For this review, take the finished solid that the model builds, in its own axes (mm). A direction names the side the tool comes from. Round coordinates to 2 decimals unless told otherwise and drop trailing zeros. Write each loop counter-clockwise with the first axis right and the second up, starting at its lowest first coordinate (ties: lowest second). Pieces come first, ordered by that corner, then holes. Notation, with made-up numbers: M -30,58 L 13,58 A20 cw 13,63 Z; hole C -40,56.5 d11. An arc over 180 degrees is marked long. Write each question's results on one line, items separated by ' | '. Start each with the question number.
```python
from build123d import *

# Parameters (mm, degrees)
SKETCH_1_W          = 250
SKETCH_1_H          = 156
SKETCH_1_W_2        = 226
SKETCH_1_H_2        = 128
EXTRUDE_1_DEPTH     = 8
SKETCH_2_W          = 235.5
SKETCH_2_H          = 139.5
CUT_EXTRUDE_3_DEPTH = 6
SKETCH_11_W         = 250
SKETCH_11_H         = 8
EXTRUDE_3_DEPTH     = 3.75
CUT_EXTRUDE_4_DEPTH = 10
SKETCH_13_R         = 1.5
CUT_EXTRUDE_5_DEPTH = 10
SKETCH_14_R         = 3
CUT_EXTRUDE_6_DEPTH = 2


with BuildPart() as part:
    # 草图1 → 凸台-拉伸1 (new body)
    with BuildSketch(Plane(origin=(0, 0, 0), x_dir=(1, 0, 0), z_dir=(0, 1, 0))):
        with Locations((25.659327926, -14.898030127)):
            Rectangle(SKETCH_1_W, SKETCH_1_H)
        with Locations((25.659327926, -14.898030127)):
            Rectangle(SKETCH_1_W_2, SKETCH_1_H_2, mode=Mode.SUBTRACT)
    extrude(amount=EXTRUDE_1_DEPTH)

    # 草图2 → 切除-拉伸3 (cut)
    with BuildSketch(Plane.XZ):
        with Locations((24.659327926, 12.898030127)):
            Rectangle(SKETCH_2_W, SKETCH_2_H)
    extrude(amount=-CUT_EXTRUDE_3_DEPTH, mode=Mode.SUBTRACT)

    # 草图11 → 凸台-拉伸3 (add)
    with BuildSketch(Plane(origin=(0, 0, -63.101969873), x_dir=(-1, 0, 0), z_dir=(0, 0, -1))):
        with Locations((-25.659327926, 4)):
            Rectangle(SKETCH_11_W, SKETCH_11_H)
    extrude(amount=EXTRUDE_3_DEPTH)

    # 草图12 → 切除-拉伸4 (cut)
    with BuildSketch(Plane.XZ):
        with BuildLine():
            Line((-89.340672074, 92.898030127), (-99.340672074, 92.898030127))
            Line((-99.340672074, 92.898030127), (-99.340672074, 82.898030127))
            ThreePointArc((-99.340672074, 82.898030127), (-96.411739886, 89.969097939), (-89.340672074, 92.898030127))
        make_face()
        with BuildLine():
            Line((-99.340672074, -56.851969873), (-99.340672074, -66.851969873))
            Line((-99.340672074, -66.851969873), (-89.340672074, -66.851969873))
            ThreePointArc((-89.340672074, -66.851969873), (-96.411739886, -63.923037684), (-99.340672074, -56.851969873))
        make_face()
        with BuildLine():
            Line((140.659327926, -66.851969873), (150.659327926, -66.851969873))
            Line((150.659327926, -66.851969873), (150.659327926, -56.851969873))
            ThreePointArc((150.659327926, -56.851969873), (147.730395738, -63.923037684), (140.659327926, -66.851969873))
        make_face()
        with BuildLine():
            Line((150.659327926, 82.898030127), (150.659327926, 92.898030127))
            Line((150.659327926, 92.898030127), (140.659327926, 92.898030127))
            ThreePointArc((140.659327926, 92.898030127), (147.730395738, 89.969097939), (150.659327926, 82.898030127))
        make_face()
    extrude(amount=-CUT_EXTRUDE_4_DEPTH, mode=Mode.SUBTRACT)

    # 草图13 → 切除-拉伸5 (cut)
    with BuildSketch(Plane.XZ):
        with Locations(Location((-86.340672074, 87.898030127, 0), (0, 0, 270))):
            Circle(SKETCH_13_R)
        with Locations(Location((137.659327926, 87.898030127, 0), (0, 0, 270))):
            Circle(SKETCH_13_R)
        with Locations(Location((137.659327926, -61.851969873, 0), (0, 0, 270))):
            Circle(SKETCH_13_R)
        with Locations(Location((-86.340672074, -61.851969873, 0), (0, 0, 270))):
            Circle(SKETCH_13_R)
    extrude(amount=-CUT_EXTRUDE_5_DEPTH, mode=Mode.SUBTRACT)

    # 草图14 → 切除-拉伸6 (cut)
    with BuildSketch(Plane(origin=(0, 8, 0), x_dir=(1, 0, 0), z_dir=(0, 1, 0))):
        with Locations(Location((-86.340672074, 61.851969873, 0), (0, 0, 270))):
            Circle(SKETCH_14_R)
        with Locations(Location((137.659327926, 61.851969873, 0), (0, 0, 270))):
            Circle(SKETCH_14_R)
        with Locations(Location((137.659327926, -87.898030127, 0), (0, 0, 270))):
            Circle(SKETCH_14_R)
        with Locations(Location((-86.340672074, -87.898030127, 0), (0, 0, 270))):
            Circle(SKETCH_14_R)
    extrude(amount=-CUT_EXTRUDE_6_DEPTH, mode=Mode.SUBTRACT)


solid = part.part
```
Item 1: We need section C-C on y = 2.75. State the section outline as (x, z) points.
Item 2: For faces 1 (the flat face through (139, 6, -63)), 2 (the flat face through (26, 8, -52)), 3 (the flat face through (23, 3, -56.852)), list the 3-axis set-ups (+Z, -Z, +X, -X, +Y, -Y) from which the entire face can be reached by the end or side of a thin tool; tool diameter is ignored.
Item 3: For probe 1 along Z at (x, y) = (137.5, 4.5); probe 2 along Z at (x, y) = (129, 3); probe 3 along X at (y, z) = (5.25, 22), list the stretches that pass through material, from the lowest coordinate up.
Item 4: We need section A-A on x = 101.5. State the section outline as (y, z) points.
Item 5: Insertion check: P1, Ø2.5, axis at x = -86.34, z = -61.85, coming from the -Y side; P2, Ø1.8, axis at x = 139, z = 89, coming from the +Y side. Each pin has a flat end and moves straight along its axis. Give the tip position at first contact, or say it passes through.
Item 6: Mouldability with a two-part tool opening along Z and no side actions: class faces 4 (the cylindrical face through (136.51, 7.01, -59.08)), 5 (the flat face through (36, 0, -58)), 6 (the cylindrical face through (-96.49, 3.94, 89.89)) as pulls with the +Z half, pulls with the -Z half, needs draft (parallel to the pull), parting line crosses it, or undercut.
Item 7: We need section B-B on z = 75.5. State the section outline as (x, y) points, then the cut area to 3 significant figures.
Numbers:
1) outline: M -99.34,-56.85 A10 ccw -89.34,-66.85 L 140.66,-66.85 A10 ccw 150.66,-56.85 L 150.66,82.9 A10 ccw 140.66,92.9 L -89.34,92.9 A10 ccw -99.34,82.9 Z; hole M -93.09,-56.85 L 142.41,-56.85 L 142.41,82.65 L -93.09,82.65 Z; hole C -86.34,-61.85 d3; hole C -86.34,87.9 d3; hole C 137.66,-61.85 d3; hole C 137.66,87.9 d3
2) face 1: +Y | face 2: +Z, -Z, +X, -X, +Y | face 3: -Y
3) probe 1: z = -66.85 to -63.34, -60.36 to -56.85, 82.65 to 86.41, 89.39 to 92.9 | probe 2: z = -66.85 to -56.85, 82.65 to 92.9 | probe 3: x = -99.34 to -93.09, 142.41 to 150.66
4) outline: M 0,-66.85 L 8,-66.85 L 8,-49.1 L 6,-49.1 L 6,-56.85 L 0,-56.85 Z; M 0,82.65 L 6,82.65 L 6,78.9 L 8,78.9 L 8,92.9 L 0,92.9 Z
5) P1: passes through | P2: stops at y = 6
6) face 4: undercut | face 5: needs draft | face 6: pulls with the +Z half
7) outline: M -99.34,0 L -93.09,0 L -93.09,6 L -87.34,6 L -87.34,8 L -99.34,8 Z; M 138.66,6 L 142.41,6 L 142.41,0 L 150.66,0 L 150.66,8 L 138.66,8 Z | area: 135 mm^2
